Here's how the part is built. I have some questions about the finished solid (model axes, mm). Face numbers are marked on the shaded views. A direction names the side the tool comes from. Give positions to 0.01 mm unless a question says otherwise; leave off trailing zeros. Write each loop counter-clockwise with the first axis right and the second up, starting at its lowest first coordinate (ties: lowest second). Pieces come first, ordered by that corner, then holes. Notation, with made-up numbers: (-23, -33) - (-11, -33) arc R30 ccw to (-11, -1) - close; hole circle Ø4 at (-17, 69.5). An arc over 180 degrees is marked (long way). One line per item, written item: value. Start each with the question number.
1) Imagine slicing it at B-B on y = 1.75. Write out the boundary of the cut face in (x, z), plus the area to 3 significant figures.
2) We'd pull the mould along X, two halves only. Please class the marked faces 3, 4 and 5: +X half, -X half, draft (parallel to the pull), parting line (faces both ways), or undercut.
3) Please list where these lines run through material, in increasing order: L1, parallel to X at y = 2.55, z = 0; L2, parallel to Y at x = 3, z = 1; L3, parallel to X at y = 12.5, z = -1.3. Write a range as [from, to].
4) I'm going to push a flat-ended pin straight in: P1, Ø1.5, axis at y = 8, z = 1, coming from the -X side. Where does the tip first touch, or does it pass through?
5) Imagine slicing it at A-A on z = 0. Write out the boundary of the cut face in (x, y), plus the area to 3 significant figures.
6) Imagine slicing it at C-C on y = 18.5. Write out the boundary of the cut face in (x, z).
7) On a 3-axis mill with a long thin cutter (end or side, diameter ignored), from which of +Z, -Z, +X, -X, +Y, -Y can I reach the whole of each face in a straight line? I mean the marked faces 1 and 2. Say none if no direction works.
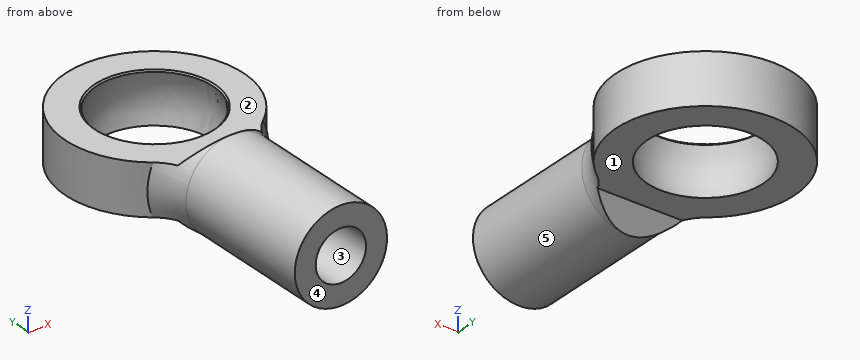
from build123d import *

# Parameters (mm, degrees)
CUT_EXTRUDE1_DEPTH      = 22.459263734
CUT_EXTRUDE1_DEPTH_BACK = 22.459263734
CUT_EXTRUDE2_DEPTH      = 21.923969522
CUT_EXTRUDE2_DEPTH_BACK = 21.923969522
SKETCH3_R               = 3
CHAMFER1_SIZE           = 0.125
CHAMFER1_SIZE2          = 0.094947636
CUT_EXTRUDE3_DEPTH      = 22.17339134
CUT_EXTRUDE3_DEPTH_BACK = 22.17339134
SKETCH7_R               = 1.5
CUT_EXTRUDE4_DEPTH      = 5


with BuildPart() as part:
    # Sketch1 → Revolve1 (revolve)
    with BuildSketch(Plane.XY, mode=Mode.PRIVATE) as revolve1_sk:
        with BuildLine():
            Line((0, 11), (0, 0))
            Line((0, 0), (2.75, 0))
            Line((2.75, 0), (2.75, 8.463651766))
            ThreePointArc((2.75, 8.463651766), (2.97496566, 9.500097013), (3.609375, 10.350010589))
            ThreePointArc((3.609375, 10.350010589), (5.151453278, 16.426792444), (0, 20))
            Line((0, 20), (0, 11))
        make_face()
    revolve(revolve1_sk.sketch.rotate(Axis((0, 0, 0), (0, -1, 0)), 90), axis=Axis((0, 0, 0), (0, -1, 0)))

    # Sketch2 → Cut-Extrude1 (cut, two sides: drawn at the far end of the back side and taken through both)
    with BuildSketch(Plane(origin=(0, 0, 0), x_dir=(0, 0, -1), z_dir=(1, 0, 0)).offset(-CUT_EXTRUDE1_DEPTH_BACK)):
        Polygon((-6.5, 9.406831178), (-2.75, 8.463651766), (-1.5, 9.406831178), (-1.5, 20.406831178), (-6.5, 20.406831178), align=None)
        Polygon((6.5, 20.406831178), (6.5, 9.406831178), (2.75, 8.463651766), (1.5, 9.406831178), (1.5, 20.406831178), align=None)
    extrude(amount=CUT_EXTRUDE1_DEPTH + CUT_EXTRUDE1_DEPTH_BACK, mode=Mode.SUBTRACT)

    # Sketch3 → Cut-Extrude2 (cut, two sides: drawn at the far end of the back side and taken through both)
    with BuildSketch(Plane.XY.offset(-CUT_EXTRUDE2_DEPTH_BACK)):
        with Locations(Location((0, 14.5, 0), (0, 0, 90))):
            Circle(SKETCH3_R)
    extrude(amount=CUT_EXTRUDE2_DEPTH + CUT_EXTRUDE2_DEPTH_BACK, mode=Mode.SUBTRACT)

    # Sketch5 → Cut-Revolve2 (revolve, cut)
    with BuildSketch(Plane.XY):
        with BuildLine():
            Line((0, 18.25), (0, 10.75))
            ThreePointArc((0, 10.75), (3.75, 14.5), (0, 18.25))
        make_face()
    revolve(axis=Axis((0, 18.25, 0), (0, -1, 0)), mode=Mode.SUBTRACT)

    # Chamfer1
    chamfer1_edges = [part.edges().sort_by_distance(p)[0] for p in [
        (0, 17.936931771, 1.5),
    ]]
    chamfer1_side = [part.faces().sort_by_distance(p)[0] for p in [
        (0, 9.555101677, 1.5),
    ]]
    chamfer(chamfer1_edges, length=CHAMFER1_SIZE, length2=CHAMFER1_SIZE2, reference=chamfer1_side[0])

    # Sketch6 → Cut-Extrude3 (cut, two sides: drawn at the far end of the back side and taken through both)
    with BuildSketch(Plane.XY.offset(1.5).offset(-CUT_EXTRUDE3_DEPTH_BACK)):
        with BuildLine():
            Line((-3.609375, 10.350010589), (-3.28292368, 10.350010589))
            ThreePointArc((-3.28292368, 10.350010589), (0, 19.791502622), (3.28292368, 10.350010589))
            Line((3.28292368, 10.350010589), (3.609375, 10.350010589))
            ThreePointArc((3.609375, 10.350010589), (0, 20), (-3.609375, 10.350010589))
        make_face()
    extrude(amount=CUT_EXTRUDE3_DEPTH + CUT_EXTRUDE3_DEPTH_BACK, mode=Mode.SUBTRACT)

    # Sketch7 → Cut-Extrude4 (cut)
    with BuildSketch(Plane.XZ):
        with Locations(Location((0, 0, 0), (0, 0, 270))):
            Circle(SKETCH7_R)
    extrude(amount=-CUT_EXTRUDE4_DEPTH, mode=Mode.SUBTRACT)


solid = part.part
Numbers:
1. outline: circle Ø5.5 at (0, 0); hole circle Ø3 at (0, 0)
1. area: 16.7 mm^2
2. face 3: undercut
2. face 4: draft
2. face 5: parting line
3. L1: [-2.75, -1.5], [1.5, 2.75]
3. L2: [9.84, 12.48], [16.52, 18.86]
3. L3: [-4.9, -2.89], [2.89, 4.9]
4. P1: x = -2.74
5. outline: (-3.61, 10.35) arc R2.5 cw to (-2.75, 8.46) - (-2.75, 0) - (-1.5, 0) - (-1.5, 5) - (1.5, 5) - (1.5, 0) - (2.75, 0) - (2.75, 8.46) arc R2.5 cw to (3.61, 10.35) - (3.28, 10.35) arc R5.29 ccw (long way) to (-3.28, 10.35) - close; hole circle Ø7.5 at (0, 14.5)
5. area: 81.6 mm^2
6. outline: (-3.46, -1.5) - (3.46, -1.5) - (3.46, 1.5) - (-3.46, 1.5) - close
7. face 1: -Z, +X, -X, +Y
7. face 2: +Z, +X, -X, +Y
